Check sheet for the modelled part. Datum: model origin and axes. Units: mm. Coordinates: 2 decimals unless noted, no trailing zeros. Loops run counter-clockwise (first coordinate to the right, second up) from the corner with the lowest first, then second, coordinate; pieces in that order, holes last. Notation, with made-up numbers: M -31,-14.5 L -10,-14.5 A18 cw -10,-4.5 Z; hole C -23.5,28 d10. An arc over 180 degrees is marked long. Answer as CSV lines item,"result". Start each with the question number.
from build123d import *

# Parameters (mm, degrees)
F0_W     = 147
F0_H     = 25
F0_R     = 4.5
F1_DEPTH = 2


with BuildPart() as f1:
    # F0 (on Front) → F1 (new body)
    with BuildSketch(Plane.XZ):
        with Locations((-1.7181, -2.911929)):
            Rectangle(F0_W, F0_H)
        with Locations((49.084206, -3.467572)):
            Circle(F0_R, mode=Mode.SUBTRACT)
        with BuildLine():
            ThreePointArc((-11.476482, -2.292731), (-10.012016, 1.242803), (-6.476482, 2.707269))
            Line((-6.476482, 2.707269), (33.523518, 2.707269))
            ThreePointArc((33.523518, 2.707269), (37.059052, 1.242803), (38.523518, -2.292731))
            ThreePointArc((38.523518, -2.292731), (37.059052, -5.828265), (33.523518, -7.292731))
            Line((33.523518, -7.292731), (-6.476482, -7.292731))
            ThreePointArc((-6.476482, -7.292731), (-10.012016, -5.828265), (-11.476482, -2.292731))
        make_face(mode=Mode.SUBTRACT)
    extrude(amount=F1_DEPTH)


solid = f1.part
Item 1: Release check for a two-part mould opening along Z. For faces 1 (the face through (53.376, -0.986, -2.116)), 2 (the face through (-3, -2, 3)) record: released by +Z, released by -Z, zero draft, split by the parting line, or undercut.
Item 2: Sectioned sample at A-A, the plane x = 22. Record the boundary of the cut face in (y, z), and give its area (3 significant figures).
Item 3: Sectioned sample at B-B, the plane z = -5.75. Record the boundary of the cut face in (x, y).
Item 4: Sectioned sample at D-D, the plane x = -9. Record the boundary of the cut face in (y, z), and give its area (3 significant figures).
Item 5: Material ranges on line 1 (X direction, y = -1.4, z = -5.5); line 2 (X direction, y = -0.3, z = -1.5); line 3 (Z direction, x = 33.5, y = -0.05), recorded low to high. Write a range as from..to.
Item 6: Sectioned sample at C-C, the plane y = -0.55. Record the boundary of the cut face in (x, z), and give its area (3 significant figures).
Item 7: Go/stop test with a flat-tipped pin: pin 1 (7 mm diameter, centred on x = 49.08, z = -3.47, fed in from +Y). Record where the tip stops, or that it passes through.
Reply:
1,face 1,"undercut"
1,face 2,"zero draft"
2,outline,"M -2,-15.41 L 0,-15.41 L 0,-7.29 L -2,-7.29 Z; M -2,2.71 L 0,2.71 L 0,9.59 L -2,9.59 Z"
2,area,"30.0 mm²"
3,outline,"M -75.22,-2 L -10.09,-2 L -10.09,0 L -75.22,0 Z; M 37.14,-2 L 45.21,-2 L 45.21,0 L 37.14,0 Z; M 52.96,-2 L 71.78,-2 L 71.78,0 L 52.96,0 Z"
4,outline,"M -2,-15.41 L 0,-15.41 L 0,-6.61 L -2,-6.61 Z; M -2,2.02 L 0,2.02 L 0,9.59 L -2,9.59 Z"
4,area,"32.7 mm²"
5,line 1,"-75.22..-10.31, 37.36..45.07, 53.1..71.78"
5,line 2,"-75.22..-11.41, 38.46..45.04, 53.13..71.78"
5,line 3,"-15.41..-7.29, 2.71..9.59"
6,outline,"M -75.22,-15.41 L 71.78,-15.41 L 71.78,9.59 L -75.22,9.59 Z; hole M -6.48,-7.29 L 33.52,-7.29 A5 ccw 33.52,2.71 L -6.48,2.71 A5 ccw Z; hole C 49.08,-3.47 d9"
6,area,"3,130 mm²"
7,pin 1,"through"
